Geometry check sheet. Reference: the model listing, model coordinates, mm. Face numbers are marked on the shaded views. A direction names the side the tool comes from. Coordinates: 2 decimals unless noted, no trailing zeros. Loops run counter-clockwise (first coordinate to the right, second up) from the corner with the lowest first, then second, coordinate; pieces in that order, holes last.
from build123d import *

# Parameters (mm, degrees)
CHAMFER1_SIZE      = 2.54
CHAMFER1_SIZE2     = 0.447870531
SKETCH3_W          = 1.27
SKETCH3_H          = 11.684
SKETCH3_W_2        = 0.896537977
SKETCH3_H_2        = 11.167643875
CUT_EXTRUDE2_DEPTH = 25.4
SKETCH4_R          = 1.783288569
CUT_EXTRUDE3_DEPTH = 32.616251091
FILLET1_R          = 0.508
SKETCH5_R          = 5.0165
SKETCH5_R_2        = 2.032
CUT_EXTRUDE4_DEPTH = 3.81


with BuildPart() as part:
    # Sketch1 → Revolve1 (revolve)
    with BuildSketch(Plane.XY, mode=Mode.PRIVATE) as revolve1_sk:
        Polygon((0, 0), (13.34752775, 0), (13.34752775, -2.248031717), (10.93452775, -2.248031717), (10.93452775, -5.296031717), (13.34752775, -5.296031717), (13.328344425, -6.6929), (12.693344425, -6.6929), (12.693344425, -8.5979), (13.328344425, -8.5979), (13.328344425, -10.16), (6.096, -10.16), (6.096, -21.844), (0, -21.844), (0, -10.16), align=None)
    revolve(revolve1_sk.sketch.rotate(Axis((0, 0, 0), (0, 1, 0)), 90), axis=Axis((0, 0, 0), (0, 1, 0)))

    # Chamfer1
    chamfer1_edges = [part.edges().sort_by_distance(p)[0] for p in [
        (0, 0, 13.34752775),
    ]]
    chamfer1_side = [part.faces().sort_by_distance(p)[0] for p in [
        (0, 0, 0),
    ]]
    chamfer(chamfer1_edges, length=CHAMFER1_SIZE, length2=CHAMFER1_SIZE2, reference=chamfer1_side[0])

    # Sketch3 → Cut-Extrude2 (cut)
    with BuildSketch(Plane.XY.offset(13.335)):
        with Locations((0, -16.002)):
            Rectangle(SKETCH3_W, SKETCH3_H)
        with Locations((5.647731012, -16.260178062)):
            Rectangle(SKETCH3_W_2, SKETCH3_H_2)
        with Locations((-5.647731012, -16.260178062)):
            Rectangle(SKETCH3_W_2, SKETCH3_H_2)
    extrude(amount=-CUT_EXTRUDE2_DEPTH, mode=Mode.SUBTRACT)

    # Sketch4 → Cut-Extrude3 (cut, through all)
    with BuildSketch(Plane(origin=(5.207, 0, 0), x_dir=(0, 0, -1), z_dir=(1, 0, 0))):
        with Locations((0, -16.034094945)):
            Circle(SKETCH4_R)
    extrude(amount=-CUT_EXTRUDE3_DEPTH, mode=Mode.SUBTRACT)

    # Fillet1
    fillet1_edges = [part.edges().sort_by_distance(p)[0] for p in [
        (5.199462023, -16.034094945, 1.783288569),
    ]]
    fillet(fillet1_edges, radius=FILLET1_R)

    # Sketch5 → Cut-Extrude4 (cut)
    with BuildSketch(Plane(origin=(0, 0, 0), x_dir=(1, 0, 0), z_dir=(0, 1, 0))):
        with Locations(Location((0, 0, 0), (0, 0, 270))):
            Circle(SKETCH5_R)
        with Locations(Location((0, 0, 0), (0, 0, 270))):
            Circle(SKETCH5_R_2, mode=Mode.SUBTRACT)
    extrude(amount=-CUT_EXTRUDE4_DEPTH, mode=Mode.SUBTRACT)


solid = part.part
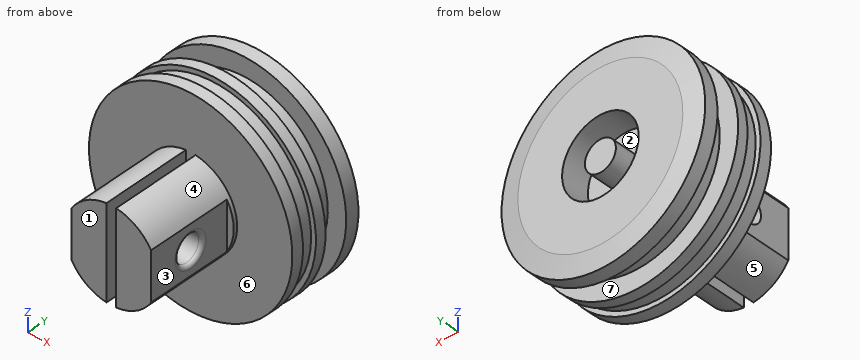
(1) Sectioned sample at B-B on y = -19.5. Record the cut outline in (x, z) (3 decimals), and give its area (3 significant figures).
Findings:
outline: (-5.199, -3.182) arc R6.096 ccw to (-0.635, -6.063) - (-0.635, 6.063) arc R6.096 ccw to (-5.199, 3.182) - close; (0.635, -6.063) arc R6.096 ccw to (5.199, -3.182) - (5.199, 3.182) arc R6.096 ccw to (0.635, 6.063) - close
area: 93.6 mm2
(2) Draft check along X on the marked faces 1, 2 and 3. Enter one of: +X half, -X half, draft (parallel to the pull), parting line (faces both ways), or undercut.
Findings:
face 1: draft
face 2: undercut
face 3: +X half
(3) Sectioned sample at D-D on y = -7.5. Record the cut outline in (x, z), and give its area (3 significant figures).
Findings:
outline: circle Ø25.39 at (0, 0)
area: 506 mm2
(4) Scan lines: L1, parallel to X at y = -18.5, z = 0.75 (3 decimals); L2, parallel to Y at x = 2, z = 0; L3, parallel to Y at x = -2.1, z = 0. Record each from-to range of solid material in increasing order.
Findings:
L1: x = -5.199 to -0.635, 0.635 to 5.199
L2: y = -21.84 to -17.82, -14.25 to 0
L3: y = -21.84 to -17.82, -14.25 to -3.81
(5) Sectioned sample at A-A on y = -1.75. Record the cut outline in (x, z).
Findings:
outline: circle Ø26.7 at (0, 0); circle Ø4.06 at (0, 0); hole circle Ø10.03 at (0, 0)
(6) Gauge pin test, flat ends, axial feed: pin 1 Ø3 at (y, z) = (-16.03, 0) entering from -X (3 decimals); pin 2 Ø4.5 at (y, z) = (-16.03, 0) entering from +X; pin 3 Ø1 at (y, z) = (-9, 2) entering from +X; pin 4 Ø6 at (x, y) = (4.5, -3.5) entering from +Z. Record the tip position at first contact, or that the pin passes through.
Findings:
pin 1: passes through
pin 2: stops at x = 5.2
pin 3: stops at x = 13.24
pin 4: stops at z = 13.23
(7) Sectioned sample at C-C on z = 0. State how many separate pieces and enclosed holes the cut face has, and give its area (3 significant figures).
Findings:
separate pieces: 3
enclosed holes: 0
area: 305 mm2
(8) Access from +Z, -Z, +X, -X, +Y, -Y to the whole of each face (thin tool, end or side, straight path). Record for the marked faces 4, 5, 6 and 7.
Findings:
face 4: +X, -Y
face 5: -X, -Y
face 6: -Y
face 7: none
